Check sheet for the modelled part. Datum: model origin and axes. Units: mm. A direction names the side the tool comes from. Give positions to 0.01 mm unless a question says otherwise; leave off trailing zeros. Loops run counter-clockwise (first coordinate to the right, second up) from the corner with the lowest first, then second, coordinate; pieces in that order, holes last. Notation, with made-up numbers: M 25,-30 L 64,-30 A4 cw 64,-26 Z; hole C -26,-26 d3. An arc over 180 degrees is marked long. Write each question's results on one line, items separated by ' | '. Start each with the question number.
1. Sectioned sample at D-D on z = 710. Record the cut outline in (x, y), and give its area (3 significant figures).
2. Sectioned sample at C-C on y = 50. Record the cut outline in (x, z).
3. Tool access check on faces 1 (the flat face through (193, 89.408, 651)), 2 (the flat face through (13.208, 38, 651)). Record the directions out of +Z, -Z, +X, -X, +Y, -Y that give a thin tool (end or side, any length) a straight path to the whole face; none if there is none.
4. Material ranges on line 1 along X through (y, z) = (85.75, 31.75); line 2 along X through (y, z) = (79, 127); line 3 along Z through (x, y) = (342, 80), recorded low to high.
5. Go/stop test with a flat-tipped pin: pin 1 (20.5 mm diameter, centred on x = 66.675, z = 127, fed in from -Y). Record where the tip stops, or that it passes through.
6. Draft check along Z on faces 3 (the flat face through (190, 78, 1320.8)), 4 (the flat face through (367.792, 39, 651)), 5 (the cylindrical face through (346.715, 82.896, 1301.164)). Enter one of: pulls with the +Z half, pulls with the -Z half, needs draft (parallel to the pull), parting line crosses it, or undercut.
7. Sectioned sample at A-A on x = 38.1. Record the cut outline in (y, z), and give its area (3 significant figures).
8. Sectioned sample at B-B on z = 1289.05. Record the cut outline in (x, y).
```python
from build123d import *

# Parameters (mm, degrees)
BOSS_EXTRUDE1_DEPTH = 1320.8
FILLET1_R           = 6.35
CUT_EXTRUDE1_REACH  = 1379.559
SKETCH2_R           = 7.9375
CUT_EXTRUDE2_REACH  = 1379.559
SKETCH3_R           = 12.7


with BuildPart() as part:
    # Sketch1 → Boss-Extrude1 (new body)
    with BuildSketch(Plane.XY):
        Polygon((367.792, 0), (381, 0), (381, 89.408), (0, 89.408), (0, 0), (13.208, 0), (13.208, 76.2), (367.792, 76.2), align=None)
    extrude(amount=BOSS_EXTRUDE1_DEPTH)

    # Fillet1
    fillet1_edges = [part.edges().sort_by_distance(p)[0] for p in [
        (367.792, 0, 660.4),
        (367.792, 76.2, 660.4),
        (13.208, 76.2, 660.4),
        (13.208, 0, 660.4),
    ]]
    fillet(fillet1_edges, radius=FILLET1_R)

    # Sketch2 → Cut-Extrude1 (cut, up to next)
    with BuildSketch(Plane(origin=(0, 89.408, 0), x_dir=(1, 0, 0), z_dir=(0, 1, 0)), mode=Mode.PRIVATE) as cut_extrude1_sk1:
        with Locations(Location((66.675, -127, 0), (0, 0, 270))):
            Circle(SKETCH2_R)
    cut_extrude1_tool1 = extrude(cut_extrude1_sk1.sketch, amount=-CUT_EXTRUDE1_REACH, mode=Mode.PRIVATE) & part.part
    # Sketch2 → Cut-Extrude1 (cut, up to next)
    with BuildSketch(Plane(origin=(0, 89.408, 0), x_dir=(1, 0, 0), z_dir=(0, 1, 0)), mode=Mode.PRIVATE) as cut_extrude1_sk2:
        with Locations(Location((314.325, -127, 0), (0, 0, 270))):
            Circle(SKETCH2_R)
    cut_extrude1_tool2 = extrude(cut_extrude1_sk2.sketch, amount=-CUT_EXTRUDE1_REACH, mode=Mode.PRIVATE) & part.part
    # Sketch2 → Cut-Extrude1 (cut, up to next)
    with BuildSketch(Plane(origin=(0, 89.408, 0), x_dir=(1, 0, 0), z_dir=(0, 1, 0)), mode=Mode.PRIVATE) as cut_extrude1_sk3:
        with Locations(Location((98.425, -444.5, 0), (0, 0, 270))):
            Circle(SKETCH2_R)
    cut_extrude1_tool3 = extrude(cut_extrude1_sk3.sketch, amount=-CUT_EXTRUDE1_REACH, mode=Mode.PRIVATE) & part.part
    # Sketch2 → Cut-Extrude1 (cut, up to next)
    with BuildSketch(Plane(origin=(0, 89.408, 0), x_dir=(1, 0, 0), z_dir=(0, 1, 0)), mode=Mode.PRIVATE) as cut_extrude1_sk4:
        with Locations(Location((282.575, -444.5, 0), (0, 0, 270))):
            Circle(SKETCH2_R)
    cut_extrude1_tool4 = extrude(cut_extrude1_sk4.sketch, amount=-CUT_EXTRUDE1_REACH, mode=Mode.PRIVATE) & part.part
    add(cut_extrude1_tool1.solids().sort_by_distance((66.675, 89.408, 127))[0], mode=Mode.SUBTRACT)
    add(cut_extrude1_tool2.solids().sort_by_distance((314.325, 89.408, 127))[0], mode=Mode.SUBTRACT)
    add(cut_extrude1_tool3.solids().sort_by_distance((98.425, 89.408, 444.5))[0], mode=Mode.SUBTRACT)
    add(cut_extrude1_tool4.solids().sort_by_distance((282.575, 89.408, 444.5))[0], mode=Mode.SUBTRACT)

    # Sketch3 → Cut-Extrude2 (cut, up to next)
    with BuildSketch(Plane(origin=(0, 89.408, 0), x_dir=(1, 0, 0), z_dir=(0, 1, 0)), mode=Mode.PRIVATE) as cut_extrude2_sk1:
        with Locations(Location((38.1, -31.75, 0), (0, 0, 270))):
            Circle(SKETCH3_R)
    cut_extrude2_tool1 = extrude(cut_extrude2_sk1.sketch, amount=-CUT_EXTRUDE2_REACH, mode=Mode.PRIVATE) & part.part
    # Sketch3 → Cut-Extrude2 (cut, up to next)
    with BuildSketch(Plane(origin=(0, 89.408, 0), x_dir=(1, 0, 0), z_dir=(0, 1, 0)), mode=Mode.PRIVATE) as cut_extrude2_sk2:
        with Locations(Location((342.9, -31.75, 0), (0, 0, 270))):
            Circle(SKETCH3_R)
    cut_extrude2_tool2 = extrude(cut_extrude2_sk2.sketch, amount=-CUT_EXTRUDE2_REACH, mode=Mode.PRIVATE) & part.part
    # Sketch3 → Cut-Extrude2 (cut, up to next)
    with BuildSketch(Plane(origin=(0, 89.408, 0), x_dir=(1, 0, 0), z_dir=(0, 1, 0)), mode=Mode.PRIVATE) as cut_extrude2_sk3:
        with Locations(Location((38.1, -1289.05, 0), (0, 0, 270))):
            Circle(SKETCH3_R)
    cut_extrude2_tool3 = extrude(cut_extrude2_sk3.sketch, amount=-CUT_EXTRUDE2_REACH, mode=Mode.PRIVATE) & part.part
    # Sketch3 → Cut-Extrude2 (cut, up to next)
    with BuildSketch(Plane(origin=(0, 89.408, 0), x_dir=(1, 0, 0), z_dir=(0, 1, 0)), mode=Mode.PRIVATE) as cut_extrude2_sk4:
        with Locations(Location((342.9, -1289.05, 0), (0, 0, 270))):
            Circle(SKETCH3_R)
    cut_extrude2_tool4 = extrude(cut_extrude2_sk4.sketch, amount=-CUT_EXTRUDE2_REACH, mode=Mode.PRIVATE) & part.part
    add(cut_extrude2_tool1.solids().sort_by_distance((38.1, 89.408, 31.75))[0], mode=Mode.SUBTRACT)
    add(cut_extrude2_tool2.solids().sort_by_distance((342.9, 89.408, 31.75))[0], mode=Mode.SUBTRACT)
    add(cut_extrude2_tool3.solids().sort_by_distance((38.1, 89.408, 1289.05))[0], mode=Mode.SUBTRACT)
    add(cut_extrude2_tool4.solids().sort_by_distance((342.9, 89.408, 1289.05))[0], mode=Mode.SUBTRACT)


solid = part.part
```
Output values:
1) outline: M 0,0 L 6.86,0 A6.35 ccw 13.21,6.35 L 13.21,69.85 A6.35 cw 19.56,76.2 L 361.44,76.2 A6.35 cw 367.79,69.85 L 367.79,6.35 A6.35 ccw 374.14,0 L 381,0 L 381,89.41 L 0,89.41 Z | area: 7,050 mm2
2) outline: M 0,0 L 13.21,0 L 13.21,1320.8 L 0,1320.8 Z; M 367.79,0 L 381,0 L 381,1320.8 L 367.79,1320.8 Z
3) face 1: +Z, -Z, +X, -X, +Y | face 2: +Z, -Z, -Y
4) line 1: 0 to 25.4, 50.8 to 330.2, 355.6 to 381 | line 2: 0 to 58.74, 74.61 to 306.39, 322.26 to 381 | line 3: 0 to 19.08, 44.42 to 1276.38, 1301.72 to 1320.8
5) pin 1: y = 76.2
6) face 3: pulls with the +Z half | face 4: needs draft | face 5: undercut
7) outline: M 76.2,0 L 89.41,0 L 89.41,19.05 L 76.2,19.05 Z; M 76.2,44.45 L 89.41,44.45 L 89.41,1276.35 L 76.2,1276.35 Z; M 76.2,1301.75 L 89.41,1301.75 L 89.41,1320.8 L 76.2,1320.8 Z | area: 16,800 mm2
8) outline: M 0,0 L 6.86,0 A6.35 ccw 13.21,6.35 L 13.21,69.85 A6.35 cw 19.56,76.2 L 25.4,76.2 L 25.4,89.41 L 0,89.41 Z; M 50.8,76.2 L 330.2,76.2 L 330.2,89.41 L 50.8,89.41 Z; M 355.6,76.2 L 361.44,76.2 A6.35 cw 367.79,69.85 L 367.79,6.35 A6.35 ccw 374.14,0 L 381,0 L 381,89.41 L 355.6,89.41 Z
